from build123d import *

# Parameters (mm, degrees)
BOSS_EXTRUDE1_DEPTH      = 75
BOSS_EXTRUDE1_DEPTH_BACK = 75
SKETCH1_W                = 20
SKETCH1_H                = 10
SKETCH3_W                = 20
SKETCH3_H                = 5
BOSS_EXTRUDE2_DEPTH      = 20
FILLET1_R                = 10
SKETCH5_W                = 20
SKETCH5_H                = 5
BOSS_EXTRUDE3_DEPTH      = 25
CHAMFER1_SIZE            = 5
CHAMFER1_SIZE_2          = 8.660254038
FILLET2_R                = 10
CUT_EXTRUDE1_DEPTH       = 101.995049384
CUT_EXTRUDE1_DEPTH_BACK  = 101.995049384
SKETCH4_R                = 2.75
CUT_EXTRUDE2_DEPTH       = 102.612007165
CUT_EXTRUDE2_DEPTH_BACK  = 2.5


# Some blends are built 0.0001 mm under size
with BuildPart() as part:
    # Sketch1 → Boss-Extrude1 (new, two sides: drawn at the far end of the back side and taken through both)
    with BuildSketch(Plane.XY.offset(-BOSS_EXTRUDE1_DEPTH_BACK)):
        Rectangle(SKETCH1_W, SKETCH1_H)
    extrude(amount=BOSS_EXTRUDE1_DEPTH + BOSS_EXTRUDE1_DEPTH_BACK)

    # Sketch3 → Boss-Extrude2 (add)
    with BuildSketch(Plane(origin=(0, 0, -75), x_dir=(-1, 0, 0), z_dir=(0, 0, -1))):
        Rectangle(SKETCH3_W, SKETCH3_H)
    extrude(amount=BOSS_EXTRUDE2_DEPTH)

    # Fillet1
    fillet1_edges = [part.edges().sort_by_distance(p)[0] for p in [
        (-10, 0, -95),
        (10, 0, -95),
    ]]
    fillet(fillet1_edges, radius=FILLET1_R - 0.0001)  # a hair under: the kernel refuses the full size

    # Sketch5 → Boss-Extrude3 (add)
    with BuildSketch(Plane.XY.offset(75)):
        with Locations((0, 5)):
            Rectangle(SKETCH5_W, SKETCH5_H)
        with Locations((0, -5)):
            Rectangle(SKETCH5_W, SKETCH5_H)
    extrude(amount=BOSS_EXTRUDE3_DEPTH)

    # Chamfer1
    # the kernel refuses this chamfer: 8.660254038, 5 mm, written as the material it adds along each edge
    with BuildSketch(Plane(origin=(10, 5, 75), x_dir=(0, -0.05789386240267149, -0.9983227437537926), z_dir=(-1, 0, 0))) as chamfer1_piece_1_section:
        Polygon((CHAMFER1_SIZE * 0.998322743754, -CHAMFER1_SIZE * 0.0578938624027), (-CHAMFER1_SIZE_2 * 0.0578938624016, -CHAMFER1_SIZE_2 * 0.998322743736), (0, 0), align=None)
    chamfer1_piece_1 = extrude(amount=20, mode=Mode.PRIVATE)
    chamfer1_piece_1 = split(chamfer1_piece_1, bisect_by=Plane(origin=(0, 7.5, 72.827003025), z_dir=(0, -1, 0)), keep=Keep.TOP, mode=Mode.PRIVATE)
    add(chamfer1_piece_1)
    with BuildSketch(Plane(origin=(-10, -5, 75), x_dir=(0, 0.05789386240267149, -0.9983227437537926), z_dir=(1, 0, 0))) as chamfer1_piece_2_section:
        Polygon((CHAMFER1_SIZE * 0.998322743754, -CHAMFER1_SIZE * 0.0578938624027), (-CHAMFER1_SIZE_2 * 0.0578938624016, -CHAMFER1_SIZE_2 * 0.998322743736), (0, 0), align=None)
    chamfer1_piece_2 = extrude(amount=20, mode=Mode.PRIVATE)
    chamfer1_piece_2 = split(chamfer1_piece_2, bisect_by=Plane(origin=(0, -7.5, 72.827003025), z_dir=(0, 1, 0)), keep=Keep.TOP, mode=Mode.PRIVATE)
    add(chamfer1_piece_2)
    # the kernel refuses this chamfer: 8.660254038, 5 mm, written as the material it takes off along each edge
    with BuildSketch(Plane(origin=(32.404819853, 5, -75), x_dir=(0, 0.019326765612700594, 0.999813220622208), z_dir=(-1, 0, 0))) as chamfer1_2_piece_1_section:
        Polygon((CHAMFER1_SIZE_2 * 0.999813220604, -CHAMFER1_SIZE_2 * 0.0193267656124), (-CHAMFER1_SIZE * 0.0193267656127, -CHAMFER1_SIZE * 0.999813220622), (0, 0), align=None)
    chamfer1_2_piece_1 = extrude(amount=64.809639706, mode=Mode.PRIVATE)
    chamfer1_2_piece_1 = split(chamfer1_2_piece_1, bisect_by=Plane(origin=(0, 2.5, -71.539331058), z_dir=(0, 1, 0)), keep=Keep.TOP, mode=Mode.PRIVATE)
    add(chamfer1_2_piece_1, mode=Mode.SUBTRACT)
    with BuildSketch(Plane(origin=(-32.404819853, -5, -75), x_dir=(0, 0.9983227437537926, -0.05789386240267045), z_dir=(1, 0, 0))) as chamfer1_2_piece_2_section:
        Polygon((CHAMFER1_SIZE * 0.998322743754, CHAMFER1_SIZE * 0.0578938624027), (-CHAMFER1_SIZE_2 * 0.0578938624016, CHAMFER1_SIZE_2 * 0.998322743736), (0, 0), align=None)
    chamfer1_2_piece_2 = extrude(amount=64.809639706, mode=Mode.PRIVATE)
    chamfer1_2_piece_2 = split(chamfer1_2_piece_2, bisect_by=Plane(origin=(0, -2.5, -71.539331058), z_dir=(0, -1, 0)), keep=Keep.TOP, mode=Mode.PRIVATE)
    add(chamfer1_2_piece_2, mode=Mode.SUBTRACT)

    # Fillet2
    fillet2_edges = [part.edges().sort_by_distance(p)[0] for p in [
        (-10, -5, 100),
        (-10, 5, 100),
        (10, -5, 100),
        (10, 5, 100),
    ]]
    fillet(fillet2_edges, radius=FILLET2_R - 0.0001)  # a hair under: the kernel refuses the full size

    # Sketch4 → Cut-Extrude1 (cut, two sides: drawn at the far end of the back side and taken through both)
    with BuildSketch(Plane(origin=(0, 2.5, 0), x_dir=(1, 0, 0), z_dir=(0, 1, 0)).offset(-CUT_EXTRUDE1_DEPTH_BACK)):
        with Locations(Location((0, 85, 0), (0, 0, 270))):
            Circle(SKETCH4_R)
        with Locations(Location((0, -90, 0), (0, 0, 270))):
            Circle(SKETCH4_R)
    extrude(amount=CUT_EXTRUDE1_DEPTH + CUT_EXTRUDE1_DEPTH_BACK, mode=Mode.SUBTRACT)

    # Sketch6 → Cut-Extrude2 (cut, two sides: drawn at the far end of the back side and taken through both)
    with BuildSketch(Plane(origin=(0, 7.5, 0), x_dir=(1, 0, 0), z_dir=(0, 1, 0)).offset(-CUT_EXTRUDE2_DEPTH_BACK)):
        Polygon((-2.38156986, -85.875), (-4.763139721, -90), (-2.38156986, -94.125), (2.38156986, -94.125), (4.763139721, -90), (2.38156986, -85.875), align=None)
    extrude(amount=CUT_EXTRUDE2_DEPTH + CUT_EXTRUDE2_DEPTH_BACK, mode=Mode.SUBTRACT)


solid = part.part
The listing builds one solid part. Answer for the finished solid, in the listing's coordinates (mm). A direction names the side the tool comes from. Give positions to 0.01 mm unless a question says otherwise; leave off trailing zeros. Order: outer loops, then holes, each group sorted by start corner. A loop starts at its lowest first (then second) coordinate and runs counter-clockwise, first axis right, second up. Notation, with made-up numbers: (62.5, 81.5) -> (68.5, 81.5) arc R34 cw to (68.5, 113.5) -> close; hole circle Ø10 at (45.25, 36). An arc over 180 degrees is marked (long way). Put each result on its own line as item: value.
Item 1: Straight lines are drawn through the part: line 1 (X direction, y = -5.45, z = 90); line 2 (Z direction, x = 0.25, y = -2.25); line 3 (Y direction, x = 7, z = 46). For each, find the intervals that lie inside material, in ascending order.
Established:
line 1: x = -10 to -2.75, 2.75 to 10
line 2: z = -95 to -87.74, -82.26 to 75
line 3: y = -5 to 5
Item 2: A cutting plane is placed at C-C on z = -53. Give the vertices of the cut face in (x, y).
Established:
outline: (-10, -5) -> (10, -5) -> (10, 5) -> (-10, 5) -> close
Item 3: For faces 1 (the face through (-7.15, 0.04, -91.99)), 2 (the face through (0, 2.5, -80)), 3 (the face through (0, 0, 75)), 4 (the face through (0, -5, 1)), determine the directions among +Z, -Z, +X, -X, +Y, -Y from which every point of the face is accessible in a straight line to the end or side of a thin tool.
Established:
face 1: -Z, -X, +Y, -Y
face 2: -Z, +X, -X, +Y
face 3: +Z, +X, -X
face 4: -Z, +X, -X, -Y
Item 4: Given P1, Ø4, axis at x = -4.5, y = 0, coming from the +Z side; P2, Ø10, axis at x = -5, z = -55.5, coming from the -Y side; P3, Ø10, axis at x = -5, z = -4.5, coming from the +Y side; P4, Ø6, axis at x = 4, z = 90.5, coming from the +Y side, each flat-ended and moving along its own axis, determine where each tip first touches the part or whether it passes through.
Established:
P1: stops at z = 75
P2: stops at y = -5
P3: stops at y = 5
P4: stops at y = 7.5
Item 5: For a pull along Z with two mould halves and no side action, classify faces 5 (the face through (-0.14, -3.73, -68.54)), 6 (the face through (0.121, 3.733, 87.253)), 7 (the face through (0, -7.5, 86)) as released by +Z, released by -Z, zero draft, split by the parting line, or undercut.
Established:
face 5: released by -Z
face 6: undercut
face 7: zero draft
Item 6: A cutting plane is placed at B-B on x = 8. Give the vertices of the cut face in (y, z).
Established:
outline: (-7.5, 71.44) -> (-5, 70) -> (-5, -66.34) -> (-2.5, -70.67) -> (-2.5, -91) -> (2.5, -91) -> (2.5, -70.67) -> (5, -66.34) -> (5, 70) -> (7.5, 71.44) -> (7.5, 96) -> (2.5, 96) -> (2.5, 75) -> (-2.5, 75) -> (-2.5, 96) -> (-7.5, 96) -> close
